Read the model definition and answer for the solid it produces. Units are mm, in the model's axes. A direction names the side the tool comes from. Coordinates: 2 decimals unless noted, no trailing zeros. Write each loop counter-clockwise with the first axis right and the second up, starting at its lowest first coordinate (ties: lowest second). Pieces come first, ordered by that corner, then holes. Notation, with made-up numbers: (46.25, 43) -> (98.25, 43) arc R27 cw to (98.25, 76) -> close; hole circle Ø11 at (-1.75, 36.5). An arc over 180 degrees is marked (long way). Return JSON: item names as keys, results as strings.
from build123d import *

# Parameters (mm, degrees)
F0_R     = 4
F1_DEPTH = 86
F2_W     = 2
F2_H     = 2.6729833462
F3_DEPTH = 86.001
F4_SIZE  = 0.5
F7_W     = 10
F7_H     = 16.0862193677
F8_DEPTH = 2.1892940191


with BuildPart() as f1:
    # F0 (on Front) → F1 (new body)
    with BuildSketch(Plane.XZ):
        Circle(F0_R)
    extrude(amount=F1_DEPTH)

    # F2 (on face) → F3 (cut, through all)
    with BuildSketch(Plane.XZ.offset(86)):
        with Locations((0, 4.0094750193)):
            Rectangle(F2_W, F2_H)
    extrude(amount=-F3_DEPTH, mode=Mode.SUBTRACT)

    # F4
    f4_edges = [f1.edges().sort_by_distance(p)[0] for p in [
        (0, -86, -4),
        (0, 0, -4),
    ]]
    chamfer(f4_edges, length=F4_SIZE)

    # F7 (on face) → F8 (cut, through all)
    with BuildSketch(Plane(origin=(2.7655894548, 0, 1.1625467594), x_dir=(0, -1, 0), z_dir=(-0.9218631516, 0, -0.3875155865))):
        with Locations((63, 0.6007021293)):
            Rectangle(F7_W, F7_H)
    extrude(amount=-F8_DEPTH, mode=Mode.SUBTRACT)


solid = f1.part
1. The part is cut by section C-C (y = -71.5). Determine the outline of the cut face in (x, z).
Taken from the geometry:
{"outline": "(-1, 2.67) -> (-1, 3.87) arc R4 ccw (long way) to (1, 3.87) -> (1, 2.67) -> close"}
2. Consider L1, parallel to X at y = -21, z = 3; L2, parallel to Z at x = -1.5, y = -38.5. Determine where each line is inside the solid, lowest interval first.
Taken from the geometry:
{"L1": "x = -2.65 to -1, 1 to 2.65", "L2": "z = -3.71 to 3.71"}
3. The part is cut by section B-B (x = 0). Determine the outline of the cut face in (y, z).
Taken from the geometry:
{"outline": "(-86, -3.5) -> (-85.5, -4) -> (-0.5, -4) -> (0, -3.5) -> (0, 2.67) -> (-86, 2.67) -> close"}
4. A tool of negligible diameter and unlimited length cuts with its end or side. For faces 1 (the face through (3, -68, 1)), 2 (the face through (0, -44, 2.673)), 3 (the face through (0, -86, 0)), from which of +Z, -Z, +X, -X, +Y, -Y can it reach the whole face along a straight path? Write none if from no direction.
Taken from the geometry:
{"face 1": "+Z, +X", "face 2": "+Z, +Y, -Y", "face 3": "+Z, -Z, +X, -X, -Y"}
5. Flat-ended cylindrical pins translate along their axes: pin 1 Ø2 at (y, z) = (-65.5, 3) entering from +X; pin 2 Ø4 at (x, y) = (-2, -23.5) entering from +Z; pin 3 Ø1.5 at (y, z) = (-67, 3) entering from +X. Find the tip coordinate at first contact, or state that the pin passes through.
Taken from the geometry:
{"pin 1": "stops at x = 2.41", "pin 2": "stops at z = 3.87", "pin 3": "stops at x = 2.31"}
6. The part is cut by section A-A (y = -61). Determine the outline of the cut face in (x, z).
Taken from the geometry:
{"outline": "(-1, 2.67) -> (-1, 3.87) arc R4 ccw (long way) to (3.79, -1.28) -> (1.74, 3.6) arc R4 ccw to (1, 3.87) -> (1, 2.67) -> close"}
